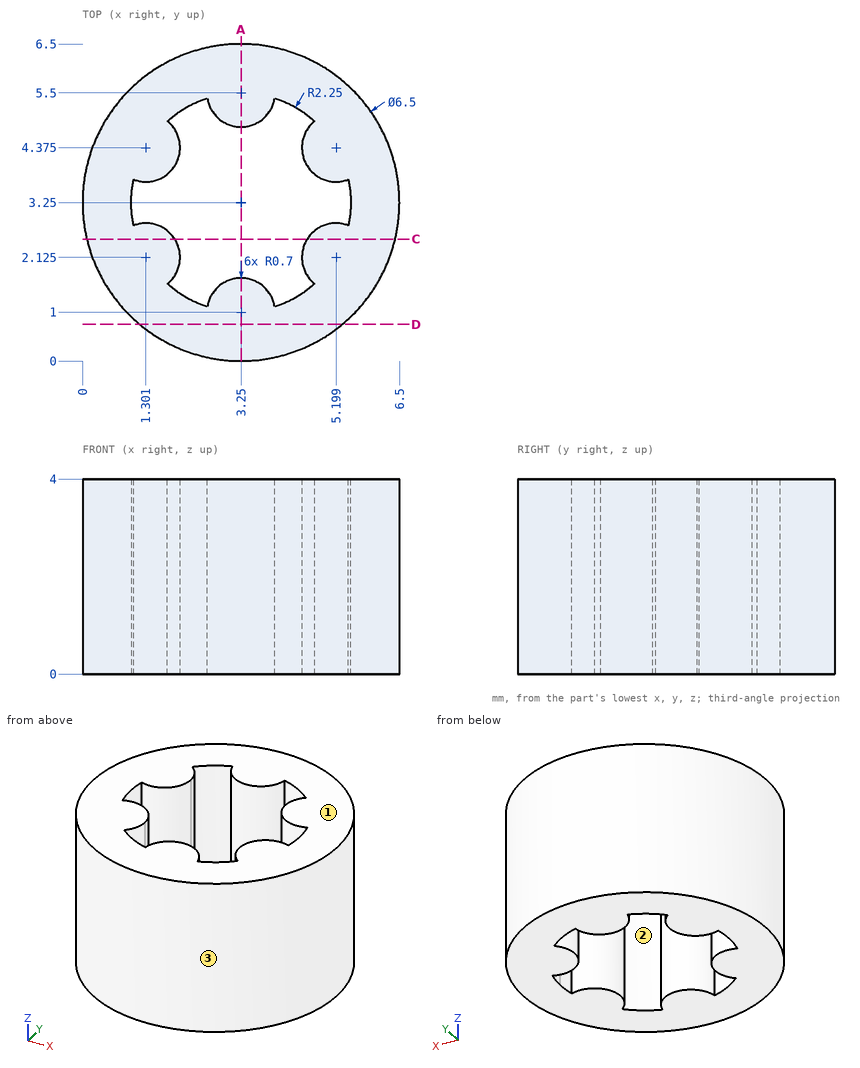
Can you work these out from the drawing? Everything is in mm from the part's minimum corner. Give positions to 0.01 mm unless a question says otherwise; leave off trailing zeros. Order: outer loops, then holes, each group sorted by start corner. A loop starts at its lowest first (then second) coordinate and runs counter-clockwise, first axis right, second up.
1. Will these pins go through, and if not, where does the flat tip stop? P1, Ø1.5, axis at x = 3.5, z = 2.5, coming from the -Y side; P2, Ø1.5, axis at y = 1.5, z = 3.5, coming from the +X side; P3, Ø1, axis at y = 5.5, z = 2, coming from the +X side; P4, Ø2, axis at y = 4.5, z = 1.5, coming from the -X side.
2. We'd pull the mould along X, two halves only. Please class the marked faces 1, 2 and 3: pulls with the +X half, pulls with the -X half, needs draft (parallel to the pull), parting line crosses it, or undercut.
3. Suppose I cut it at D-D (y = 0.75). List the corners of the cut face in (x, z) for me.
4. I need wall thicknesses on L1, parallel to Y at x = 3.25, z = 0.3; L2, parallel to X at y = 6.25, z = 2.55 (1 decimal); L3, parallel to Y at x = 4, z = 0.8. Which ranges of each line are inside material? Lowest first, please.
5. Suppose I cut it at A-A (x = 3.25). List the corners of the cut face in (y, z) for me, plus the area to 3 significant figures.
6. Suppose I cut it at C-C (y = 2.5). List the corners of the cut face in (x, z) for me.
Solved:
1. P1: stops at y = 0
1. P2: stops at x = 6.34
1. P3: stops at x = 5.99
1. P4: stops at x = 0.01
2. face 1: needs draft
2. face 2: undercut
2. face 3: parting line crosses it
3. outline: (1.17, 0) - (5.33, 0) - (5.33, 4) - (1.17, 4) - close
4. L1: y = 0 to 1.7, 4.8 to 6.5
4. L2: x = 2 to 4.5
4. L3: y = 0.09 to 1.13, 5.37 to 6.41
5. outline: (0, 0) - (1.7, 0) - (1.7, 4) - (0, 4) - close; (4.8, 0) - (6.5, 0) - (6.5, 4) - (4.8, 4) - close
5. area: 13.6 mm2
6. outline: (0.09, 0) - (1.89, 0) - (1.89, 4) - (0.09, 4) - close; (4.61, 0) - (6.41, 0) - (6.41, 4) - (4.61, 4) - close
